For this review, take the finished solid that the model builds, in its own axes (mm). A direction names the side the tool comes from. Give positions to 0.01 mm unless a question says otherwise; leave off trailing zeros. Write each loop counter-clockwise with the first axis right and the second up, starting at its lowest first coordinate (ties: lowest second). Pieces come first, ordered by that corner, then holes. Notation, with made-up numbers: (-16, 82) -> (1, 82) arc R19 cw to (1, 103) -> close; hole circle Ø4 at (-35.5, -28.5). An arc over 180 degrees is marked (long way). Write item = value, one per line.
```python
from build123d import *

# Parameters (mm, degrees)
SKETCH1_R           = 1.6
SKETCH1_R_2         = 5.5
SKETCH1_R_3         = 2.55
BOSS_EXTRUDE1_DEPTH = 3
SKETCH2_R           = 8.025
CUT_EXTRUDE1_DEPTH  = 2


with BuildPart() as part:
    # Sketch1 → Boss-Extrude1 (new body)
    with BuildSketch(Plane(origin=(0, 0, 0), x_dir=(1, 0, 0), z_dir=(0, 1, 0))):
        with BuildLine():
            Line((35, -32.5), (-35, -32.5))
            ThreePointArc((-35, -32.5), (-38.535533906, -31.035533906), (-40, -27.5))
            Line((-40, -27.5), (-40, 14.306951673))
            ThreePointArc((-40, 14.306951673), (-39.448126611, 17.081406557), (-37.876524164, 19.433475836))
            Line((-37.876524164, 19.433475836), (-20.438099577, 36.871900423))
            ThreePointArc((-20.438099577, 36.871900423), (-16.973258212, 39.187033407), (-12.886199154, 40))
            Line((-12.886199154, 40), (12.886199154, 40))
            ThreePointArc((12.886199154, 40), (16.973258212, 39.187033407), (20.438099577, 36.871900423))
            Line((20.438099577, 36.871900423), (37.876524164, 19.433475836))
            ThreePointArc((37.876524164, 19.433475836), (39.448126611, 17.081406557), (40, 14.306951673))
            Line((40, 14.306951673), (40, -27.5))
            ThreePointArc((40, -27.5), (38.535533906, -31.035533906), (35, -32.5))
        make_face()
        with Locations((21.920310217, 0)):
            Circle(SKETCH1_R, mode=Mode.SUBTRACT)
        with Locations((-21.920310217, 0)):
            Circle(SKETCH1_R, mode=Mode.SUBTRACT)
        Circle(SKETCH1_R_2, mode=Mode.SUBTRACT)
        with Locations((0, 21.920310217)):
            Circle(SKETCH1_R, mode=Mode.SUBTRACT)
        with Locations((-33.333013665, 0)):
            Circle(SKETCH1_R_3, mode=Mode.SUBTRACT)
        with Locations((0, 33.333013665)):
            Circle(SKETCH1_R_3, mode=Mode.SUBTRACT)
        with Locations((33.333013665, 0)):
            Circle(SKETCH1_R_3, mode=Mode.SUBTRACT)
        with BuildLine():
            Line((27.45, -24.9), (27.45, -16.2))
            ThreePointArc((27.45, -16.2), (30, -13.65), (32.55, -16.2))
            Line((32.55, -16.2), (32.55, -24.9))
            ThreePointArc((32.55, -24.9), (30, -27.45), (27.45, -24.9))
        make_face(mode=Mode.SUBTRACT)
        with BuildLine():
            Line((17.45, -24.9), (17.45, -16.2))
            ThreePointArc((17.45, -16.2), (20, -13.65), (22.55, -16.2))
            Line((22.55, -16.2), (22.55, -24.9))
            ThreePointArc((22.55, -24.9), (20, -27.45), (17.45, -24.9))
        make_face(mode=Mode.SUBTRACT)
        with BuildLine():
            Line((7.45, -24.9), (7.45, -16.2))
            ThreePointArc((7.45, -16.2), (10, -13.65), (12.55, -16.2))
            Line((12.55, -16.2), (12.55, -24.9))
            ThreePointArc((12.55, -24.9), (10, -27.45), (7.45, -24.9))
        make_face(mode=Mode.SUBTRACT)
        with BuildLine():
            Line((-2.55, -24.9), (-2.55, -16.2))
            ThreePointArc((-2.55, -16.2), (0, -13.65), (2.55, -16.2))
            Line((2.55, -16.2), (2.55, -24.9))
            ThreePointArc((2.55, -24.9), (0, -27.45), (-2.55, -24.9))
        make_face(mode=Mode.SUBTRACT)
        with BuildLine():
            Line((-12.55, -24.9), (-12.55, -16.2))
            ThreePointArc((-12.55, -16.2), (-10, -13.65), (-7.45, -16.2))
            Line((-7.45, -16.2), (-7.45, -24.9))
            ThreePointArc((-7.45, -24.9), (-10, -27.45), (-12.55, -24.9))
        make_face(mode=Mode.SUBTRACT)
        with BuildLine():
            Line((-22.55, -24.9), (-22.55, -16.2))
            ThreePointArc((-22.55, -16.2), (-20, -13.65), (-17.45, -16.2))
            Line((-17.45, -16.2), (-17.45, -24.9))
            ThreePointArc((-17.45, -24.9), (-20, -27.45), (-22.55, -24.9))
        make_face(mode=Mode.SUBTRACT)
        with BuildLine():
            Line((-32.55, -24.9), (-32.55, -16.2))
            ThreePointArc((-32.55, -16.2), (-30, -13.65), (-27.45, -16.2))
            Line((-27.45, -16.2), (-27.45, -24.9))
            ThreePointArc((-27.45, -24.9), (-30, -27.45), (-32.55, -24.9))
        make_face(mode=Mode.SUBTRACT)
    extrude(amount=BOSS_EXTRUDE1_DEPTH)

    # Sketch2 → Cut-Extrude1 (cut)
    with BuildSketch(Plane(origin=(0, 3, 0), x_dir=(1, 0, 0), z_dir=(0, 1, 0))):
        Circle(SKETCH2_R)
    extrude(amount=-CUT_EXTRUDE1_DEPTH, mode=Mode.SUBTRACT)


solid = part.part
```
(1) To check wall thickness, follow probe 1 along Z at (x, y) = (0, 1.1) (3 decimals); probe 2 along X at (y, z) = (0.5, 0); probe 3 along X at (y, z) = (1.6, 0) (3 decimals). State the ranges of each line that lie inside material, in increasing order.
Answers below:
probe_1 = -40 to -35.883, -30.783 to -23.52, -20.32 to -8.025, 8.025 to 13.65, 27.45 to 32.5
probe_2 = -40 to -35.88, -30.78 to -23.52, -20.32 to -5.5, 5.5 to 20.32, 23.52 to 30.78, 35.88 to 40
probe_3 = -40 to -35.883, -30.783 to -23.52, -20.32 to -8.025, 8.025 to 20.32, 23.52 to 30.783, 35.883 to 40
(2) Take a section at D-D (x = 29). Write out the cut boundary in (y, z), plus the area to 3 significant figures.
Answers below:
outline = (0, -28.31) -> (3, -28.31) -> (3, 13.85) -> (0, 13.85) -> close; (0, 27.25) -> (3, 27.25) -> (3, 32.5) -> (0, 32.5) -> close
area = 142 mm^2
(3) Tool access review of faces 1 (the face through (12.55, 1, 20)), 2 (the face through (-40, 1, 7)): name each direction out of +Z, -Z, +X, -X, +Y, -Y from which nothing blocks a thin tool from reaching the whole face with its end or side.
Answers below:
face_1 = +Y, -Y
face_2 = +Z, -Z, -X, +Y, -Y
(4) Take a section at B-B (x = -10). Write out the cut boundary in (y, z), plus the area to 3 significant figures.
Answers below:
outline = (0, -40) -> (3, -40) -> (3, 13.65) -> (0, 13.65) -> close; (0, 27.45) -> (3, 27.45) -> (3, 32.5) -> (0, 32.5) -> close
area = 176 mm^2
(5) Take a section at C-C (x = 0). Write out the cut boundary in (y, z) (3 decimals), plus the area to 3 significant figures.
Answers below:
outline = (0, -40) -> (3, -40) -> (3, -35.883) -> (0, -35.883) -> close; (0, -30.783) -> (3, -30.783) -> (3, -23.52) -> (0, -23.52) -> close; (0, -20.32) -> (3, -20.32) -> (3, -8.025) -> (1, -8.025) -> (1, -5.5) -> (0, -5.5) -> close; (0, 5.5) -> (1, 5.5) -> (1, 8.025) -> (3, 8.025) -> (3, 13.65) -> (0, 13.65) -> close; (0, 27.45) -> (3, 27.45) -> (3, 32.5) -> (0, 32.5) -> close
area = 108 mm^2
(6) For pin 1 (1.9 mm diameter, centred on x = -21.92, z = 0, fed in from +Y); pin 2 (14.5 mm diameter, centred on x = 0, z = 0, fed in from +Y), all flat-tipped, find the tip position at first contact; note any pin that passes through.
Answers below:
pin_1 = through
pin_2 = 1
(7) Take a section at A-A (z = 0). Write out the cut boundary in (x, y) (3 decimals), plus the area to 3 significant figures.
Answers below:
outline = (-40, 0) -> (-35.883, 0) -> (-35.883, 3) -> (-40, 3) -> close; (-30.783, 0) -> (-23.52, 0) -> (-23.52, 3) -> (-30.783, 3) -> close; (-20.32, 0) -> (-5.5, 0) -> (-5.5, 1) -> (-8.025, 1) -> (-8.025, 3) -> (-20.32, 3) -> close; (5.5, 0) -> (20.32, 0) -> (20.32, 3) -> (8.025, 3) -> (8.025, 1) -> (5.5, 1) -> close; (23.52, 0) -> (30.783, 0) -> (30.783, 3) -> (23.52, 3) -> close; (35.883, 0) -> (40, 0) -> (40, 3) -> (35.883, 3) -> close
area = 147 mm^2
